Verification items for the finished model (mm, model axes). Give positions to 0.01 mm unless a question says otherwise; leave off trailing zeros. Order: outer loops, then holes, each group sorted by start corner. A loop starts at its lowest first (then second) coordinate and runs counter-clockwise, first axis right, second up. Notation, with made-up numbers: (77, 32) - (97, 32) arc R15 ccw to (97, 59) - close; hole circle Ø5 at (62, -7.75). An arc over 180 degrees is marked (long way). Answer as a JSON object with one key per item and string values. Group by question number.
(1) Section check C-C (y = 5.75). Record the boundary of the cut face in (x, z) (3 decimals), then the cut area to 3 significant figures.
(2) Section check A-A (z = 0). Record the boundary of the cut face in (x, y) (3 decimals), then the cut area to 3 significant figures.
(3) Depth check by flat-ended pin: pin 1 Ø1.5 at (x, y) = (-1, 3) entering from -Z; pin 2 Ø1 at (y, z) = (2.5, 1.5) entering from -X. Enter the tip coordinate at first touch or a pass-through.
(4) Thickness scan on line 1 (X direction, y = 5.25, z = 0) (3 decimals); line 2 (Z direction, x = 1.25, y = 5.25). Record the ranges inside material, lowest first.
(5) Section check B-B (x = 0). Record the boundary of the cut face in (y, z) (3 decimals).
(6) Mould release check, pull along Z, two halves, no side actions. Record for faces 1 (the face through (3.233, 3.944, 1.341)), 2 (the face through (-0.3, 4.05, 1.34)), 3 (the face through (0, 8, 2)): +Z half, -Z half, draft (parallel to the pull), parting line (faces both ways), or undercut.
(7) Section check D-D (z = 2). Record the boundary of the cut face in (x, y).
```python
from build123d import *

# Parameters (mm, degrees)
SKETCH1_R           = 3.5
BOSS_EXTRUDE1_DEPTH = 8
SKETCH2_R           = 1.375
CUT_EXTRUDE1_DEPTH  = 8
FILLET1_R           = 0.125


with BuildPart() as part:
    # Sketch1 → Boss-Extrude1 (new body)
    with BuildSketch(Plane(origin=(0, 0, 0), x_dir=(1, 0, 0), z_dir=(0, 1, 0))):
        Circle(SKETCH1_R)
    extrude(amount=BOSS_EXTRUDE1_DEPTH)

    # Sketch2 → Cut-Extrude1 (cut)
    with BuildSketch(Plane(origin=(0, 8, 0), x_dir=(1, 0, 0), z_dir=(0, 1, 0))):
        Circle(SKETCH2_R)
    extrude(amount=-CUT_EXTRUDE1_DEPTH, mode=Mode.SUBTRACT)

    # Fillet1
    fillet1_edges = [part.edges().sort_by_distance(p)[0] for p in [
        (-1.375, 0, 0),
        (-1.375, 8, 0),
    ]]
    fillet(fillet1_edges, radius=FILLET1_R)


solid = part.part
```
Solutions:
{
 "1": {"outline": "circle Ø7 at (0, 0); hole circle Ø2.75 at (0, 0)", "area": "32.5 mm2"},
 "2": {"outline": "(-3.5, 0) - (-1.5, 0) arc R0.125 ccw to (-1.375, 0.125) - (-1.375, 7.875) arc R0.125 ccw to (-1.5, 8) - (-3.5, 8) - close; (1.375, 0.125) arc R0.125 ccw to (1.5, 0) - (3.5, 0) - (3.5, 8) - (1.5, 8) arc R0.125 ccw to (1.375, 7.875) - close", "area": "34.0 mm2"},
 "3": {"pin 1": "stops at z = -3.49", "pin 2": "stops at x = -3.35"},
 "4": {"line 1": "x = -3.5 to -1.375, 1.375 to 3.5", "line 2": "z = -3.27 to -0.57, 0.57 to 3.27"},
 "5": {"outline": "(0, -3.5) - (8, -3.5) - (8, -1.5) arc R0.125 ccw to (7.875, -1.375) - (0.125, -1.375) arc R0.125 ccw to (0, -1.5) - close; (0, 1.5) arc R0.125 ccw to (0.125, 1.375) - (7.875, 1.375) arc R0.125 ccw to (8, 1.5) - (8, 3.5) - (0, 3.5) - close"},
 "6": {"face 1": "parting line", "face 2": "undercut", "face 3": "draft"},
 "7": {"outline": "(-2.87, 0) - (2.87, 0) - (2.87, 8) - (-2.87, 8) - close"}
}
